```python
from build123d import *

# Parameters (mm, degrees)
F0_R          = 10
F1_DEPTH      = 2
F1_DEPTH_BACK = 2
F3_D          = 6
F4_SIZE       = 0.5
F7_DEPTH      = 4.001


# Not quite as in the source:
# - two fillets or chamfers of one size are made in one step


with BuildPart() as f1:
    # F0 (on Front) → F1 (new body, two sides)
    with BuildSketch(Plane.XZ) as f1_sk:
        with BuildLine():
            ThreePointArc((10.4685027699, 13.3944186047), (8.0122088596, 16.6160342353), (7.4491243619, 20.6279069767))
            ThreePointArc((7.4491243619, 20.6279069767), (5.6031552573, 26.4854439284), (0, 29))
            ThreePointArc((0, 29), (-5.6031552573, 26.4854439284), (-7.4491243619, 20.6279069767))
            ThreePointArc((-7.4491243619, 20.6279069767), (-8.0122088596, 16.6160342353), (-10.4685027699, 13.3944186047))
            ThreePointArc((-10.4685027699, 13.3944186047), (-14.7224318643, 8.5), (-16.8341581655, 2.368780036))
            ThreePointArc((-16.8341581655, 2.368780036), (-18.3960121877, -1.3692407048), (-21.5888536497, -3.862822555))
            ThreePointArc((-21.5888536497, -3.862822555), (-25.7386449011, -8.39024717), (-25.1147367097, -14.5))
            ThreePointArc((-25.1147367097, -14.5), (-20.1354896438, -18.0951967583), (-14.1397292878, -16.7650844217))
            ThreePointArc((-14.1397292878, -16.7650844217), (-10.3838033281, -15.2467935304), (-6.3656553956, -15.7631986406))
            ThreePointArc((-6.3656553956, -15.7631986406), (0, -17), (6.3656553956, -15.7631986406))
            ThreePointArc((6.3656553956, -15.7631986406), (10.3838033281, -15.2467935304), (14.1397292878, -16.7650844217))
            ThreePointArc((14.1397292878, -16.7650844217), (20.1354896438, -18.0951967583), (25.1147367097, -14.5))
            ThreePointArc((25.1147367097, -14.5), (25.7386449011, -8.39024717), (21.5888536497, -3.862822555))
            ThreePointArc((21.5888536497, -3.862822555), (18.3960121877, -1.3692407048), (16.8341581655, 2.368780036))
            ThreePointArc((16.8341581655, 2.368780036), (14.7224318643, 8.5), (10.4685027699, 13.3944186047))
        make_face()
        Circle(F0_R, mode=Mode.SUBTRACT)
    extrude(amount=F1_DEPTH)
    extrude(f1_sk.sketch, amount=-F1_DEPTH_BACK)

    # F3 (through all)
    with Locations(Plane.XZ.offset(2)):
        with Locations((0, 21.5), (-18.6195461814, -10.75), (18.6195461814, -10.75)):
            Hole(F3_D / 2)

    # F4
    f4_edges = [f1.edges().sort_by_distance(p)[0] for p in [
        (-10, -2, 0),
        (10, 0, 0),
        (-10, 2, 0),
        (8.012209, -2, 16.616034),
        (8.012209, 2, 16.616034),
        (14.722432, -2, 8.5),
        (14.722432, 2, 8.5),
        (0, -2, 29),
        (18.396012, -2, -1.369241),
        (-8.012209, -2, 16.616034),
        (25.114737, -2, -14.5),
        (-14.722432, -2, 8.5),
        (10.383803, -2, -15.246794),
        (-18.396012, -2, -1.369241),
        (0, -2, -17),
        (-25.114737, -2, -14.5),
        (-10.383803, -2, -15.246794),
        (0, 2, 29),
        (18.396012, 2, -1.369241),
        (-8.012209, 2, 16.616034),
        (25.114737, 2, -14.5),
        (-14.722432, 2, 8.5),
        (10.383803, 2, -15.246794),
        (-18.396012, 2, -1.369241),
        (0, 2, -17),
        (-25.114737, 2, -14.5),
        (-10.383803, 2, -15.246794),
    ]]
    chamfer(f4_edges, length=F4_SIZE)

    # F6 (on face) → F7 (cut, through all)
    with BuildSketch(Plane(origin=(0, 2, 0), x_dir=(-1, 0, 0), z_dir=(0, 1, 0))):
        with BuildLine():
            ThreePointArc((-2, 9.7979589711), (0, 10), (2, 9.7979589711))
            Line((2, 9.7979589711), (2, 12))
            ThreePointArc((2, 12), (0, 14), (-2, 12))
            Line((-2, 12), (-2, 9.7979589711))
        make_face()
        with BuildLine():
            Line((-9.3923048454, -7.7320508076), (-7.4852813742, -6.6310302931))
            ThreePointArc((-7.4852813742, -6.6310302931), (-8.6602540378, -5), (-9.4852813742, -3.166928678))
            Line((-9.4852813742, -3.166928678), (-11.3923048454, -4.2679491924))
            ThreePointArc((-11.3923048454, -4.2679491924), (-12.124355653, -7), (-9.3923048454, -7.7320508076))
        make_face()
        with BuildLine():
            Line((11.3923048454, -4.2679491924), (9.4852813742, -3.166928678))
            ThreePointArc((9.4852813742, -3.166928678), (8.6602540378, -5), (7.4852813742, -6.6310302931))
            Line((7.4852813742, -6.6310302931), (9.3923048454, -7.7320508076))
            ThreePointArc((9.3923048454, -7.7320508076), (12.124355653, -7), (11.3923048454, -4.2679491924))
        make_face()
    extrude(amount=-F7_DEPTH, mode=Mode.SUBTRACT)


solid = f1.part
```
Can you work these out from the model? Positions are in its coordinate system, mm. A direction names the side the tool comes from. Coordinates: 2 decimals unless noted, no trailing zeros. Loops run counter-clockwise (first coordinate to the right, second up) from the corner with the lowest first, then second, coordinate; pieces in that order, holes last.
Item 1: Suppose I cut it at B-B (x = 0). Please give me the cut outline in (y, z).
Answers below:
outline: (-2, -16.5) - (-1.5, -17) - (1.5, -17) - (2, -16.5) - (2, -10.5) - (1.5, -10) - (-1.5, -10) - (-2, -10.5) - close; (-2, 14) - (2, 14) - (2, 18.5) - (-2, 18.5) - close; (-2, 24.5) - (2, 24.5) - (2, 28.5) - (1.5, 29) - (-1.5, 29) - (-2, 28.5) - close
Item 2: Which directions (+Z, -Z, +X, -X, +Y, -Y) give clear straight access to the entire face, cutting with the end or side of a thin tool? Please do faces 4 (the face through (15, 0, 8)), 5 (the face through (8.838, -1.635, 4.962)), 6 (the face through (-8.6, 0, 5.1)).
Answers below:
face 4: +Z, +X, +Y, -Y
face 5: -Y
face 6: +Y, -Y
Item 3: If we mould it in two halves opening along X, with no side actions, what happens to faces 1 (the face through (-14.677, -0.021, 8.579)), 2 (the face through (5, -2, -10)), 3 (the face through (21.617, 0.028, -10.618))? For each: released by +X, released by -X, zero draft, split by the parting line, or undercut.
Answers below:
face 1: released by -X
face 2: zero draft
face 3: undercut
Item 4: I'm going to push flat-ended pins straight in: pin 1 (1 mm diameter, centred on y = -1, z = 4.5, fed in from -X); pin 2 (1 mm diameter, centred on x = -8.5, y = 0, fed in from +Z); pin 3 (1.5 mm diameter, centred on y = 0.5, z = 19, fed in from -X); pin 4 (9.5 mm diameter, centred on x = 18.62, z = -10.75, fed in from -Y). Where does each tip first touch, or does it pass through?
Answers below:
pin 1: stops at x = -16.52
pin 2: stops at z = 16.65
pin 3: stops at x = -7.53
pin 4: stops at y = -2
Item 5: Suppose I cut it at A-A (z = 21.5). Please give me the cut outline in (x, y), then the cut area to 3 significant figures.
Answers below:
outline: (-7.5, -1.5) - (-7, -2) - (-3, -2) - (-3, 2) - (-7, 2) - (-7.5, 1.5) - close; (3, -2) - (7, -2) - (7.5, -1.5) - (7.5, 1.5) - (7, 2) - (3, 2) - close
area: 35.5 mm2
Item 6: Please list where these lines run through material, in increasing order: L1, parallel to Z at x = 0, y = 0.4; L2, parallel to X at y = -0.15, z = -6.5; L3, parallel to X at y = 0.8, z = 11.
Answers below:
L1: z = -17 to -10, 14 to 18.5, 24.5 to 29
L2: x = -24.8 to -12.33, 12.33 to 24.8
L3: x = -12.96 to -2, 2 to 12.96
Item 7: Suppose I cut it at C-C (y = 0.75). Please give me the cut outline in (x, z).
Answers below:
outline: (-21.59, -3.86) arc R7.5 ccw (long way) to (-14.14, -16.77) arc R8 cw to (-6.37, -15.76) arc R17 ccw to (6.37, -15.76) arc R8 cw to (14.14, -16.77) arc R7.5 ccw (long way) to (21.59, -3.86) arc R8 cw to (16.83, 2.37) arc R17 ccw to (10.47, 13.39) arc R8 cw to (7.45, 20.63) arc R7.5 ccw (long way) to (-7.45, 20.63) arc R8 cw to (-10.47, 13.39) arc R17 ccw to (-16.83, 2.37) arc R8 cw to start; hole circle Ø6 at (-18.62, -10.75); hole (-11.39, -4.27) arc R2 ccw to (-9.39, -7.73) - (-7.49, -6.63) arc R10 ccw to (7.49, -6.63) - (9.39, -7.73) arc R2 ccw to (11.39, -4.27) - (9.49, -3.17) arc R10 ccw to (2, 9.8) - (2, 12) arc R2 ccw to (-2, 12) - (-2, 9.8) arc R10 ccw to (-9.49, -3.17) - close; hole circle Ø6 at (0, 21.5); hole circle Ø6 at (18.62, -10.75)
